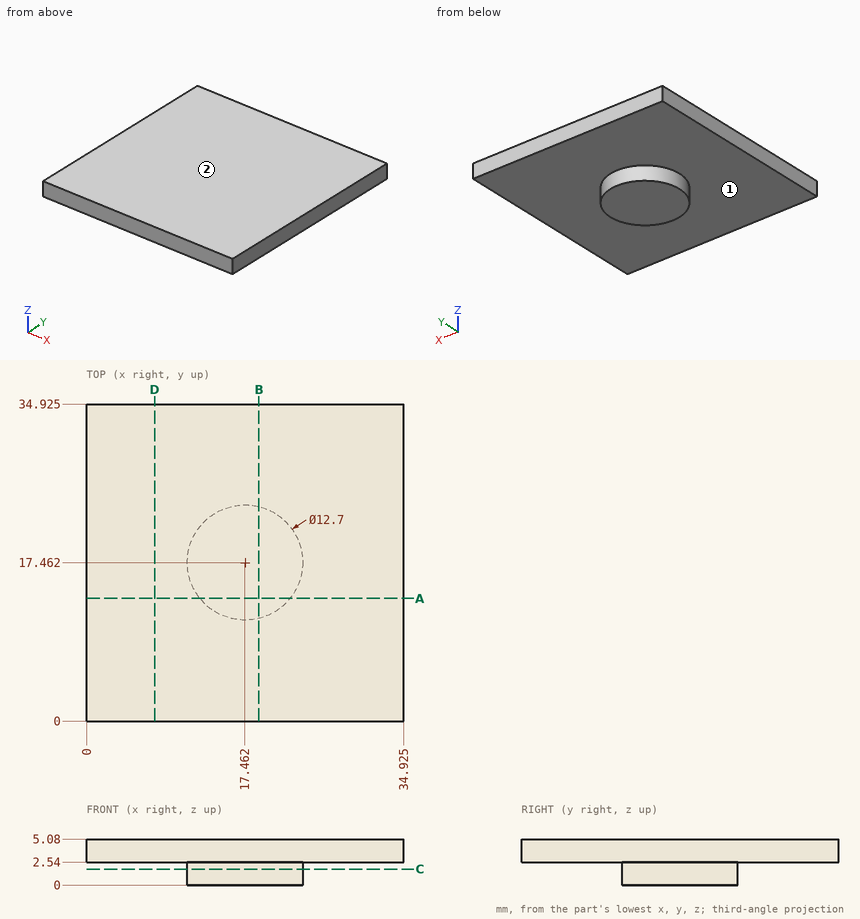
Print and shaded views of the part. All mm, measured from the part's lowest x, y and z. A direction names the side the tool comes from. Give positions to 0.01 mm unless a question says otherwise; leave off trailing zeros. Loops run counter-clockwise (first coordinate to the right, second up) from the corner with the lowest first, then second, coordinate; pieces in that order, holes last. Notation, with made-up numbers: M 72.25,12.5 L 97.25,12.5 A9 cw 97.25,25.5 Z; hole C 71.5,-38 d6. An arc over 180 degrees is marked long. Write each question's results on one line, items separated by ' | '.
Q1. Band-saw the part on B-B on x = 19. Write the cut outline in (y, z) (1 decimal).
Geometry check:
outline: M 0,2.5 L 11.3,2.5 L 11.3,0 L 23.6,0 L 23.6,2.5 L 34.9,2.5 L 34.9,5.1 L 0,5.1 Z
Q2. Flat gauge pins, fed straight in: P1, Ø1.5, axis at y = 12, z = 4, coming from the -X side; P2, Ø1, axis at x = 8.5, y = 12, coming from the -Z side. Where does each tip first touch, or does it go through?
Geometry check:
P1: stops at x = 0 | P2: stops at z = 2.54
Q3. Band-saw the part on C-C on z = 1.75. Write the cut outline in (x, y), and give its area (3 significant figures).
Geometry check:
outline: C 17.46,17.46 d12.7 | area: 127 mm²
Q4. Probe probe 1 along Z at (x, y) = (5, 22); probe 2 along X at (y, z) = (13, 1.45) (1 decimal); probe 3 along Y at (x, z) = (22, 2.2) (1 decimal). List the from-to ranges inside material, lowest first.
Geometry check:
probe 1: z = 2.54 to 5.08 | probe 2: x = 12.9 to 22 | probe 3: y = 13 to 21.9
Q5. Band-saw the part on A-A on y = 13.5. Write the cut outline in (x, z) (1 decimal), and give its area (3 significant figures).
Geometry check:
outline: M 0,2.5 L 12.5,2.5 L 12.5,0 L 22.4,0 L 22.4,2.5 L 34.9,2.5 L 34.9,5.1 L 0,5.1 Z | area: 114 mm²
Q6. Which spindle directions (+Z, -Z, +X, -X, +Y, -Y) get a long thin tool onto all of the face, cutting with end or side? Do the marked faces 1 and 2. Say none if no direction does.
Geometry check:
face 1: -Z | face 2: +Z, +X, -X, +Y, -Y
Q7. Band-saw the part on D-D on x = 7.5. Write the cut outline in (y, z) (1 decimal).
Geometry check:
outline: M 0,2.5 L 34.9,2.5 L 34.9,5.1 L 0,5.1 Z
